Source: CAD feature listing. Evaluate the final solid. Frame: model axes, mm. A direction names the side the tool comes from. Round coordinates to 2 decimals unless told otherwise and drop trailing zeros. Loops run counter-clockwise (first coordinate to the right, second up) from the corner with the lowest first, then second, coordinate; pieces in that order, holes last.
(1) Mould query, pull axis Y, two halves, no side actions, for faces 1 (the flat face through (28, 14, 4)), 2 (the flat face through (33, 0, -5.5)), 3 (the flat face through (27.5, -3, 0)). Classes: pulls with the +Y half, pulls with the -Y half, needs draft (parallel to the pull), parting line crosses it, or undercut.
(2) Section D-D, the plane y = -8. Return the cut outline in (x, z).
(3) Section A-A, the plane y = 0. Return the cut outline in (x, z).
(4) Section B-B, the plane x = 5.5. Return the cut outline in (y, z), plus the area to 3 significant figures.
(5) Section C-C, the plane z = 4.5. Return the cut outline in (x, y).
(6) Material intervals for probe 1 along X at (y, z) = (0, 3.25); probe 2 along Z at (x, y) = (34.5, 0); probe 3 along X at (y, z) = (10, 12.5), sorted ascending.
(7) First-contact query: pin 1 Ø14 at (x, y) = (11, -5.5) entering from -Z; pin 2 Ø8 at (x, y) = (17.5, 8) entering from +Z; pin 3 Ø3 at (x, z) = (6.5, -0.5) entering from -Y. Flat tips, straight axial feed; report the tip coordinate or a pass-through.
(8) Set-up query: faces 4 (the flat face through (14, 0, 9)), 5 (the flat face through (14, 0, 0)), 6 (the flat face through (22, 9, 4)), 7 (the cylindrical face through (3.759, -10.435, 4.437)), 8 (the cylindrical face through (32.57, 2.74, 8.8)). Return all of +Z, -Z, +X, -X, +Y, -Y with unobstructed straight access to the full face (end or side cutting, diameter ignored); none if empty.
Autodesk Fusion 360 part; units mm, degrees
sketch "Sketch1" plane through (0, 0, 0) normal (0, 1, 0) x (1, 0, 0)
  line L0 (0, 0) -> (15, 0)
  line L1 (15, 0) -> (15, -9)
  line L2 (15, -9) -> (0, -9)
  line L3 (0, -9) -> (0, 0)
  line L4 (15, -9) -> (17.5, -9)
  line L5 (17.5, 0) -> (15, 0)
  line L6 (17.5, -9) -> (17.5, 0)
  line L7 (17.5, -9) -> (27.5, -9)
  line L8 (27.5, -9) -> (27.5, -14.5)
  line L9 (27.5, -14.5) -> (37.5, -14.5)
  line L10 (37.5, -14.5) -> (37.5, 5.5)
  line L11 (37.5, 5.5) -> (27.5, 5.5)
  line L12 (27.5, 5.5) -> (27.5, 0)
  line L13 (27.5, 0) -> (17.5, 0)
  line L14 (27.5, -9) -> (27.5, 0)
  dimension "d1" = 15
  dimension "d2" = 9
  dimension "d3" = 15
  dimension "d55" = 10
  dimension "d56" = 5.5
  dimension "d57" = 10
  dimension "d58" = 20
extrude "Extrude2" add sketch "Sketch1" along normal mid plane 28 contours L0 L1 L2 L3 | L1 L4 L5 L6
fillet "Fillet1" radius 12.5 2 edges at (0, -14, 4.5) (0, 14, 4.5)
sketch "Sketch2" plane through (0, 0, 9) normal (0, 0, 1) x (-1, 0, 0)
  line L0 (-12.5, 14) -> (-17.5, 14)
  line L1 (-17.5, -14) -> (-12.5, -14)
  line L2 (0, 0) -> (-7.5, 0) construction
  circle A0 centre (-7.5, 0) radius 2.6
  arc A1 (-12.5, -14) -> (0, -1.5) centre (-12.5, -1.5) ccw
  line L3 (-17.5, 14) -> (-17.5, -14)
  line L4 (0, -1.5) -> (0, 1.5)
  arc A2 (0, 1.5) -> (-12.5, 14) centre (-12.5, 1.5) ccw
  dimension "d28" = 7.5
  dimension "d29" = 5.2
extrude "Extrude4" cut sketch "Sketch2" against normal through all contours A0
extrude "Extrude9" add sketch "Sketch1" against normal blind 5 from surface at 14 contours L6 L7 L13 L14
extrude "Extrude10" add sketch "Sketch1" along normal blind 5 from surface at -14 contours L6 L7 L13 L14
extrude "Extrude11" add sketch "Sketch1" along normal mid plane 28 contours L8 L9 L10 L11 L12 L14
sketch "Sketch4" plane through (37.5, 0, 0) normal (1, 0, 0) x (0, 1, 0)
  line L0 (-14, -5.5) -> (14, -5.5)
  line L1 (14, -5.5) -> (14, 14.5)
  line L2 (14, 14.5) -> (-14, 14.5)
  line L3 (-14, 14.5) -> (-14, -5.5)
  line L4 (0, 14.5) -> (0, 4.5) construction
  line L5 (0, 4.5) -> (-14, 4.5) construction
  circle A0 centre (0, 4.5) radius 5.1
  dimension "d67" = 10
  dimension "d68" = 10.2
extrude "Extrude12" cut sketch "Sketch4" against normal blind 10 contours A0
equation "d27 = ( 25 / 2 ) * 1 mm"
equation "d56 = ( ( 20 - 9 ) / 2 ) * 1 mm"
equation "d59 = ( 28 / 2 ) * 1 mm"
equation "d62 = ( -28 / 2 ) * 1 mm"
equation "d67 = ( 20 / 2 ) * 1 mm"
Output values:
1. face 1: pulls with the +Y half
1. face 2: needs draft
1. face 3: undercut
2. outline: (1.82, 0) - (17.5, 0) - (17.5, 9) - (1.82, 9) - close; (27.5, -5.5) - (37.5, -5.5) - (37.5, 14.5) - (27.5, 14.5) - close
3. outline: (0, 0) - (4.9, 0) - (4.9, 9) - (0, 9) - close; (10.1, 0) - (17.5, 0) - (17.5, 9) - (10.1, 9) - close; (27.5, -5.5) - (37.5, -5.5) - (37.5, -0.6) - (27.5, -0.6) - close; (27.5, 9.6) - (37.5, 9.6) - (37.5, 14.5) - (27.5, 14.5) - close
4. outline: (-11.86, 0) - (-1.66, 0) - (-1.66, 9) - (-11.86, 9) - close; (1.66, 0) - (11.86, 0) - (11.86, 9) - (1.66, 9) - close
4. area: 184 mm2
5. outline: (0, -1.5) arc R12.5 ccw to (12.5, -14) - (37.5, -14) - (37.5, -5.1) - (27.5, -5.1) - (27.5, -9) - (17.5, -9) - (17.5, 9) - (27.5, 9) - (27.5, 5.1) - (37.5, 5.1) - (37.5, 14) - (12.5, 14) arc R12.5 ccw to (0, 1.5) - close; hole circle Ø5.2 at (7.5, 0)
6. probe 1: x = 0 to 4.9, 10.1 to 17.5
6. probe 2: z = -5.5 to -0.6, 9.6 to 14.5
6. probe 3: x = 27.5 to 37.5
7. pin 1: stops at z = 0
7. pin 2: stops at z = 9
7. pin 3: stops at y = -13.13
8. face 4: +Z, -X, +Y, -Y
8. face 5: -Z, -X, +Y, -Y
8. face 6: +Z, -Z
8. face 7: +Z, -Z, -X, -Y
8. face 8: +X
